```python
from build123d import *

# Parameters (mm, degrees)
SKETCH2_R           = 8.5
BOSS_EXTRUDE1_DEPTH = 4
SKETCH3_W           = 12
SKETCH3_H           = 9
CUT_EXTRUDE1_DEPTH  = 2
FILLET1_R           = 3.5
SKETCH4_R           = 3.725
SKETCH4_R_2         = 0.75
CUT_EXTRUDE2_DEPTH  = 13.186057607


with BuildPart() as part:
    # Sketch2 → Boss-Extrude1 (new body)
    with BuildSketch(Plane(origin=(0, 0, 0), x_dir=(1, 0, 0), z_dir=(0, 1, 0))):
        with Locations(Location((0, 0, 0), (0, 0, 270))):
            Circle(SKETCH2_R)
    extrude(amount=BOSS_EXTRUDE1_DEPTH)

    # Sketch3 → Cut-Extrude1 (cut)
    with BuildSketch(Plane(origin=(0, 4, 0), x_dir=(1, 0, 0), z_dir=(0, 1, 0))):
        Rectangle(SKETCH3_W, SKETCH3_H)
    extrude(amount=-CUT_EXTRUDE1_DEPTH, mode=Mode.SUBTRACT)

    # Fillet1
    fillet1_edges = [part.edges().sort_by_distance(p)[0] for p in [
        (6, 3, -4.5),
        (6, 3, 4.5),
        (-6, 3, 4.5),
        (-6, 3, -4.5),
    ]]
    fillet(fillet1_edges, radius=FILLET1_R)

    # Sketch4 → Cut-Extrude2 (cut, through all)
    with BuildSketch(Plane(origin=(0, 2, 0), x_dir=(1, 0, 0), z_dir=(0, 1, 0))):
        with Locations(Location((0, 0, 0), (0, 0, 270))):
            Circle(SKETCH4_R)
        with Locations(Location((-4.977045146, 0.478562033, 0), (0, 0, 270))):
            Circle(SKETCH4_R_2)
        with Locations(Location((4.977045146, 0.478562033, 0), (0, 0, 90))):
            Circle(SKETCH4_R_2)
    extrude(amount=-CUT_EXTRUDE2_DEPTH, mode=Mode.SUBTRACT)


solid = part.part
```
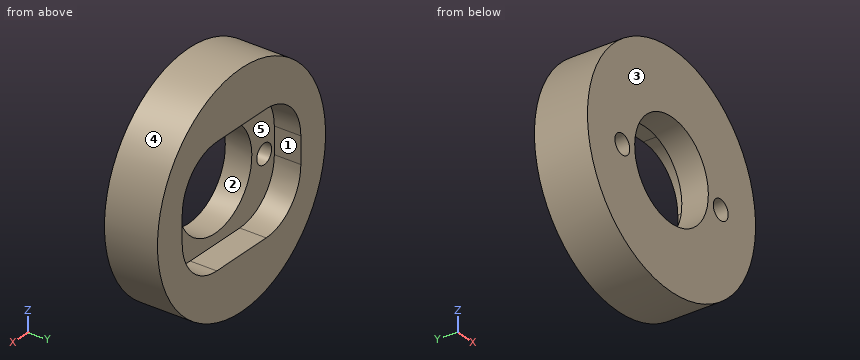
Can you work these out from the model? Positions are in its coordinate system, mm. Face numbers are marked on the shaded views. A direction names the side the tool comes from. Coordinates: 2 decimals unless noted, no trailing zeros. Write each loop counter-clockwise with the first axis right and the second up, starting at its lowest first coordinate (ties: lowest second). Pieces come first, ordered by that corner, then holes. Notation, with made-up numbers: (46, 52.25) - (67, 52.25) arc R24 ccw to (67, 67.25) - close; hole circle Ø11 at (88.25, 0.5). An arc over 180 degrees is marked (long way). Return JSON: item names as keys, results as strings.
Q1. If we section it at B-B (y = 2.8): Please give me the cut outline in (x, z).
Computed values:
{"outline": "circle Ø17 at (0, 0); hole (-6, -1) arc R3.5 ccw to (-2.5, -4.5) - (2.5, -4.5) arc R3.5 ccw to (6, -1) - (6, 1) arc R3.5 ccw to (2.5, 4.5) - (-2.5, 4.5) arc R3.5 ccw to (-6, 1) - close"}
Q2. I'm going to push flat-ended pins straight in: pin 1 Ø4.5 at (x, z) = (2.5, 1) entering from +Y; pin 2 Ø2 at (x, z) = (-1, -0.5) entering from -Y; pin 3 Ø1.6 at (x, y) = (1, 3) entering from -Z; pin 4 Ø1 at (y, z) = (0.5, -2.5) entering from +X. Where does each tip first touch, or does it pass through?
Computed values:
{"pin 1": "stops at y = 2", "pin 2": "passes through", "pin 3": "stops at z = -8.5", "pin 4": "stops at x = 8.26"}
Q3. Please list where these lines run through material, in increasing order: L1, parallel to X at y = 1.2, z = 0 (3 decimals); L2, parallel to X at y = 1.5, z = -0.75; L3, parallel to Z at x = 0.75, y = 3.05. Write a range as from..to.
Computed values:
{"L1": "x = -8.5..-5.555, -4.4..-3.725, 3.725..4.4, 5.555..8.5", "L2": "x = -8.47..-5.68, -4.28..-3.65, 3.65..4.28, 5.68..8.47", "L3": "z = -8.47..-4.5, 4.5..8.47"}
Q4. If we section it at C-C (z = 0): Please give me the cut outline in (x, y) (3 decimals).
Computed values:
{"outline": "(-8.5, 0) - (-5.555, 0) - (-5.555, 2) - (-6, 2) - (-6, 4) - (-8.5, 4) - close; (-4.4, 0) - (-3.725, 0) - (-3.725, 2) - (-4.4, 2) - close; (3.725, 0) - (4.4, 0) - (4.4, 2) - (3.725, 2) - close; (5.555, 0) - (8.5, 0) - (8.5, 4) - (6, 4) - (6, 2) - (5.555, 2) - close"}
Q5. If we section it at D-D (z = 2.25): Please give me the cut outline in (x, y).
Computed values:
{"outline": "(-8.2, 0) - (-2.97, 0) - (-2.97, 2) - (-5.77, 2) - (-5.77, 4) - (-8.2, 4) - close; (2.97, 0) - (8.2, 0) - (8.2, 4) - (5.77, 4) - (5.77, 2) - (2.97, 2) - close"}
Q6. Thinking about a two-plate mould opening in Z: for the marked faces 3, 4 and 5, which applies, +Z half, -Z half, draft (parallel to the pull), parting line (faces both ways), or undercut?
Computed values:
{"face 3": "draft", "face 4": "parting line", "face 5": "undercut"}
Q7. If we section it at A-A (x = 0): Please give me the cut outline in (y, z) (3 decimals).
Computed values:
{"outline": "(0, -8.5) - (4, -8.5) - (4, -4.5) - (2, -4.5) - (2, -3.725) - (0, -3.725) - close; (0, 3.725) - (2, 3.725) - (2, 4.5) - (4, 4.5) - (4, 8.5) - (0, 8.5) - close"}
Q8. On a 3-axis mill with a long thin cutter (end or side, diameter ignored), from which of +Z, -Z, +X, -X, +Y, -Y can I reach the whole of each face in a straight line? I mean the marked faces 1 and 2. Say none if no direction works.
Computed values:
{"face 1": "+Y", "face 2": "+Y, -Y"}
